from build123d import *

# Parameters (mm, degrees)
SKETCH1_W                        = 156
SKETCH1_H                        = 260
BOSS_EXTRUDE1_DEPTH              = 10
BOSS_EXTRUDE2_DEPTH              = 66
SKETCH3_R                        = 40
CUT_EXTRUDE1_DEPTH               = 77
SKETCH4_W                        = 20
SKETCH4_H                        = 37.5
CUT_EXTRUDE2_DEPTH               = 5
SKETCH6_W                        = 15
SKETCH6_H                        = 15
BOSS_EXTRUDE3_DEPTH              = 10
SKETCH7_R                        = 4
CUT_EXTRUDE4_DEPTH               = 10
FILLET1_R                        = 2
SKETCH8_W                        = 156
SKETCH8_H                        = 10
BOSS_EXTRUDE4_DEPTH              = 10
SKETCH9_R                        = 4
CUT_EXTRUDE5_DEPTH               = 77
SKETCH10_W                       = 156
SKETCH10_H                       = 10
BOSS_EXTRUDE5_DEPTH              = 25
SKETCH11_W                       = 28
SKETCH11_H                       = 295
BOSS_EXTRUDE6_DEPTH              = 10
BOSS_EXTRUDE7_DEPTH              = 212
SKETCH13_R                       = 3
CUT_EXTRUDE6_DEPTH               = 11
BOSS_EXTRUDE10_DEPTH             = 212
SKETCH18_R                       = 3
CUT_EXTRUDE8_DEPTH               = 11
SKETCH19_R                       = 10
CUT_EXTRUDE9_DEPTH               = 113
BOSS_EXTRUDE11_REACH             = 47.35
SKETCH20_W                       = 10
SKETCH20_H                       = 86
BOSS_EXTRUDE11_DIRECTION_2_REACH = 366.652
FILLET2_R                        = 20
SKETCH21_R                       = 15
CUT_EXTRUDE11_DEPTH              = 5
SKETCH22_W                       = 30
SKETCH22_H                       = 20
CUT_EXTRUDE12_DEPTH              = 1
CUT_EXTRUDE12_DEPTH_BACK         = 213
SKETCH23_W                       = 40
SKETCH23_H                       = 6.35
CUT_EXTRUDE13_DEPTH              = 1
CUT_EXTRUDE13_DEPTH_BACK         = 213


with BuildPart() as part:
    # Sketch1 → Boss-Extrude1 (new body)
    with BuildSketch(Plane(origin=(0, 0, 0), x_dir=(1, 0, 0), z_dir=(0, 1, 0))):
        Rectangle(SKETCH1_W, SKETCH1_H)
    extrude(amount=BOSS_EXTRUDE1_DEPTH)

    # Sketch2 → Boss-Extrude2 (add)
    with BuildSketch(Plane.XZ):
        Polygon((-73, -120), (-73, 125), (73, 125), (73, -120), (78, -120), (78, 130), (-78, 130), (-78, -120), align=None)
    extrude(amount=BOSS_EXTRUDE2_DEPTH)

    # Sketch3 → Cut-Extrude1 (cut, through all)
    with BuildSketch(Plane(origin=(0, 10, 0), x_dir=(1, 0, 0), z_dir=(0, 1, 0))):
        with Locations((0, -70)):
            Circle(SKETCH3_R)
    extrude(amount=-CUT_EXTRUDE1_DEPTH, mode=Mode.SUBTRACT)

    # Sketch4 → Cut-Extrude2 (cut)
    with BuildSketch(Plane.XY.offset(130)):
        with Locations((-62.5, -47.25)):
            Rectangle(SKETCH4_W, SKETCH4_H)
        with Locations((62.5, -47.25)):
            Rectangle(SKETCH4_W, SKETCH4_H)
    extrude(amount=-CUT_EXTRUDE2_DEPTH, mode=Mode.SUBTRACT)

    # Sketch6 → Boss-Extrude3 (add)
    with BuildSketch(Plane.XZ.offset(66)):
        with Locations((0, 137.5)):
            Rectangle(SKETCH6_W, SKETCH6_H)
    extrude(amount=-BOSS_EXTRUDE3_DEPTH)

    # Sketch7 → Cut-Extrude4 (cut)
    with BuildSketch(Plane.XZ.offset(66)):
        with Locations((0, 137.5)):
            Circle(SKETCH7_R)
    extrude(amount=-CUT_EXTRUDE4_DEPTH, mode=Mode.SUBTRACT)

    # Fillet1
    fillet1_edges = [part.edges().sort_by_distance(p)[0] for p in [
        (7.5, -61, 145),
        (-7.5, -61, 145),
    ]]
    fillet(fillet1_edges, radius=FILLET1_R)

    # Sketch8 → Boss-Extrude4 (add)
    with BuildSketch(Plane(origin=(0, 0, -130), x_dir=(-1, 0, 0), z_dir=(0, 0, -1))):
        with Locations((0, 5)):
            Rectangle(SKETCH8_W, SKETCH8_H)
    extrude(amount=BOSS_EXTRUDE4_DEPTH)

    # Sketch9 → Cut-Extrude5 (cut, through all)
    with BuildSketch(Plane(origin=(0, 10, 0), x_dir=(1, 0, 0), z_dir=(0, 1, 0))):
        with Locations((-68, 130)):
            Circle(SKETCH9_R)
        with Locations((68, 130)):
            Circle(SKETCH9_R)
    extrude(amount=-CUT_EXTRUDE5_DEPTH, mode=Mode.SUBTRACT)

    # Sketch10 → Boss-Extrude5 (add)
    with BuildSketch(Plane(origin=(0, 0, -140), x_dir=(-1, 0, 0), z_dir=(0, 0, -1))):
        with Locations((0, 5)):
            Rectangle(SKETCH10_W, SKETCH10_H)
    extrude(amount=BOSS_EXTRUDE5_DEPTH)

    # Sketch11 → Boss-Extrude6 (add)
    with BuildSketch(Plane(origin=(0, 10, 0), x_dir=(1, 0, 0), z_dir=(0, 1, 0))):
        with Locations((-92, 17.5)):
            Rectangle(SKETCH11_W, SKETCH11_H)
        with Locations((92, 17.5)):
            Rectangle(SKETCH11_W, SKETCH11_H)
    extrude(amount=-BOSS_EXTRUDE6_DEPTH)

    # Sketch12 → Boss-Extrude7 (add)
    with BuildSketch(Plane.ZY.offset(106)):
        Polygon((-165, 0), (-190.349999035, -86), (-210.349999035, -86), (-210.349999035, -76), (-190.349999035, -76), (-165, 10), align=None)
    extrude(amount=-BOSS_EXTRUDE7_DEPTH)

    # Sketch13 → Cut-Extrude6 (cut, through all)
    with BuildSketch(Plane(origin=(0, -76, 0), x_dir=(1, 0, 0), z_dir=(0, 1, 0))):
        with Locations((-96, 200.349999035)):
            Circle(SKETCH13_R)
        with Locations((96, 200.349999035)):
            Circle(SKETCH13_R)
    extrude(amount=-CUT_EXTRUDE6_DEPTH, mode=Mode.SUBTRACT)

    # Sketch17 → Boss-Extrude10 (add)
    with BuildSketch(Plane(origin=(106, 0, 0), x_dir=(0, 0, -1), z_dir=(1, 0, 0))):
        Polygon((-130, 0), (-179.65212315, -86), (-199.65212315, -86), (-199.65212315, -76), (-179.65212315, -76), (-130, 10), align=None)
    extrude(amount=-BOSS_EXTRUDE10_DEPTH)

    # Sketch18 → Cut-Extrude8 (cut, through all)
    with BuildSketch(Plane(origin=(0, -76, 0), x_dir=(1, 0, 0), z_dir=(0, 1, 0))):
        with Locations((-96, -189.65212315)):
            Circle(SKETCH18_R)
        with Locations((96, -189.65212315)):
            Circle(SKETCH18_R)
    extrude(amount=-CUT_EXTRUDE8_DEPTH, mode=Mode.SUBTRACT)

    # Sketch19 → Cut-Extrude9 (cut)
    with BuildSketch(Plane.XY.offset(130)):
        with Locations((-62.5, -38.5)):
            Circle(SKETCH19_R)
        with Locations((62.5, -38.5)):
            Circle(SKETCH19_R)
    extrude(amount=CUT_EXTRUDE9_DEPTH, mode=Mode.SUBTRACT)

    # Boss-Extrude11: up to this face of the body (flat: up to its plane)
    boss_extrude11_end = Plane(part.part.faces().sort_by_distance((0, -33, -177.674999518))[0])
    # Sketch20 → Boss-Extrude11 (add, up to the picked face)
    with BuildSketch(Plane(origin=(0, 0, -165), x_dir=(-1, 0, 0), z_dir=(0, 0, -1)), mode=Mode.PRIVATE) as boss_extrude11_sk1:
        with Locations((-101, -43)):
            Rectangle(SKETCH20_W, SKETCH20_H)
    boss_extrude11_tool1 = split(extrude(boss_extrude11_sk1.sketch, amount=BOSS_EXTRUDE11_REACH, mode=Mode.PRIVATE), bisect_by=boss_extrude11_end, keep=Keep.BOTH, mode=Mode.PRIVATE)
    add(boss_extrude11_tool1.solids().sort_by_distance((101, -43, -165))[0])
    # Sketch20 → Boss-Extrude11 (add, up to the picked face)
    with BuildSketch(Plane(origin=(0, 0, -165), x_dir=(-1, 0, 0), z_dir=(0, 0, -1)), mode=Mode.PRIVATE) as boss_extrude11_sk2:
        with Locations((101, -43)):
            Rectangle(SKETCH20_W, SKETCH20_H)
    boss_extrude11_tool2 = split(extrude(boss_extrude11_sk2.sketch, amount=BOSS_EXTRUDE11_REACH, mode=Mode.PRIVATE), bisect_by=boss_extrude11_end, keep=Keep.BOTH, mode=Mode.PRIVATE)
    add(boss_extrude11_tool2.solids().sort_by_distance((-101, -43, -165))[0])

    # Sketch20 → Boss-Extrude11 direction 2 (add, up to next)
    with BuildSketch(Plane(origin=(0, 0, -165), x_dir=(-1, 0, 0), z_dir=(0, 0, -1)), mode=Mode.PRIVATE) as boss_extrude11_direction_2_sk1:
        with Locations((-101, -43)):
            Rectangle(SKETCH20_W, SKETCH20_H)
    boss_extrude11_direction_2_tool1 = extrude(boss_extrude11_direction_2_sk1.sketch, amount=-BOSS_EXTRUDE11_DIRECTION_2_REACH, mode=Mode.PRIVATE) - part.part
    add(boss_extrude11_direction_2_tool1.solids().sort_by_distance((101, -43, -165))[0])
    # Sketch20 → Boss-Extrude11 direction 2 (add, up to next)
    with BuildSketch(Plane(origin=(0, 0, -165), x_dir=(-1, 0, 0), z_dir=(0, 0, -1)), mode=Mode.PRIVATE) as boss_extrude11_direction_2_sk2:
        with Locations((101, -43)):
            Rectangle(SKETCH20_W, SKETCH20_H)
    boss_extrude11_direction_2_tool2 = extrude(boss_extrude11_direction_2_sk2.sketch, amount=-BOSS_EXTRUDE11_DIRECTION_2_REACH, mode=Mode.PRIVATE) - part.part
    add(boss_extrude11_direction_2_tool2.solids().sort_by_distance((-101, -43, -165))[0])

    # Fillet2
    fillet2_edges = [part.edges().sort_by_distance(p)[0] for p in [
        (0, 10, -165),
        (0, 10, 130),
    ]]
    fillet(fillet2_edges, radius=FILLET2_R)

    # Sketch21 → Cut-Extrude11 (cut)
    with BuildSketch(Plane(origin=(78, 0, 0), x_dir=(0, 0, -1), z_dir=(1, 0, 0))):
        with Locations((90, -30.5)):
            Circle(SKETCH21_R)
    extrude(amount=-CUT_EXTRUDE11_DEPTH, mode=Mode.SUBTRACT)

    # Sketch22 → Cut-Extrude12 (cut, two sides)
    with BuildSketch(Plane(origin=(106, 0, 0), x_dir=(0, 0, -1), z_dir=(1, 0, 0))) as cut_extrude12_sk:
        with Locations((-105, -76)):
            Rectangle(SKETCH22_W, SKETCH22_H)
        with Locations((49.5, -76)):
            Rectangle(SKETCH22_W, SKETCH22_H)
    extrude(amount=CUT_EXTRUDE12_DEPTH, mode=Mode.SUBTRACT)
    extrude(cut_extrude12_sk.sketch, amount=-CUT_EXTRUDE12_DEPTH_BACK, mode=Mode.SUBTRACT)

    # Sketch23 → Cut-Extrude13 (cut, two sides)
    with BuildSketch(Plane.ZY.offset(106)) as cut_extrude13_sk:
        with Locations((-102.849999035, -82.825)):
            Rectangle(SKETCH23_W, SKETCH23_H)
        with Locations((92.150000965, -82.825)):
            Rectangle(SKETCH23_W, SKETCH23_H)
    extrude(amount=CUT_EXTRUDE13_DEPTH, mode=Mode.SUBTRACT)
    extrude(cut_extrude13_sk.sketch, amount=-CUT_EXTRUDE13_DEPTH_BACK, mode=Mode.SUBTRACT)


solid = part.part
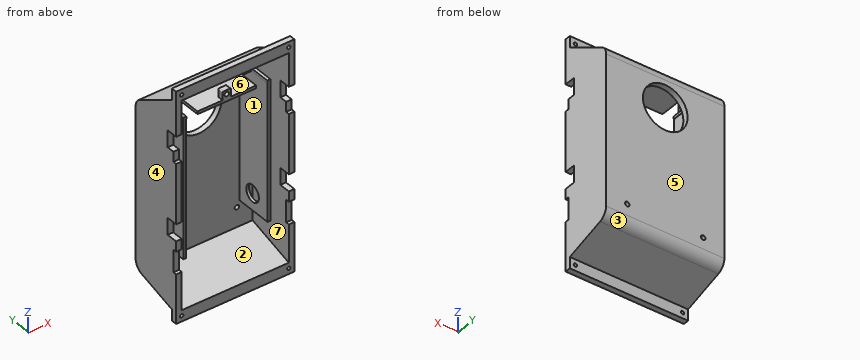
CAD build for the part. Positions are in the model's coordinates, mm. Face numbers are marked on the shaded views. A direction names the side the tool comes from. Give positions to 0.01 mm unless a question says otherwise; leave off trailing zeros. Write each loop counter-clockwise with the first axis right and the second up, starting at its lowest first coordinate (ties: lowest second). Pieces come first, ordered by that corner, then holes. Notation, with made-up numbers: (48, -27) - (81, -27) arc R10 ccw to (81, -12) - close; hole circle Ø3 at (17, 53). An arc over 180 degrees is marked (long way). Answer as CSV lines item,"result".
Q1. Drill centre lines: line 1 (X direction, y = -55, z = -8.5); line 2 (Z direction, x = -75.5, y = -47); line 3 (X direction, y = -61, z = 137). Where is each one in solid material? Low to high. Write a range as from..to.
Result set:
line 1,"-106..-96, -78..-73, 73..78, 96..106"
line 2,"-181.8..-178.85, -120..130, 157.14..162.91"
line 3,"-106..-96, -7.5..-3.97, 3.97..7.5, 96..106"
Q2. Flat gauge pins, fed straight in: pin 1 Ø8 at (x, z) = (99.5, 112) entering from -Y; pin 2 Ø3 at (x, z) = (48.5, -154.5) entering from +Y; pin 3 Ø18 at (x, y) = (62.5, -38.5) entering from -Z. Where does each tip first touch, or does it go through?
Result set:
pin 1,"y = -66"
pin 2,"y = 9.78"
pin 3,"z = -181.95"
Q3. Band-saw the part on D-D (z = -25). Give the cut face in (x, y), and give its area (3 significant figures).
Result set:
outline,"(-106, -86) - (-96, -86) - (-96, 0) - (-78, 0) - (-78, -66) - (-73, -66) - (-73, 0) - (73, 0) - (73, -66) - (78, -66) - (78, 0) - (96, 0) - (96, -86) - (106, -86) - (106, 10) - (-106, 10) - close"
area,"4,500 mm²"
Q4. Pull direction X, two halves, no side cores. Call the marked faces 1, 2, 3 and 4: released by +X, released by -X, zero draft, split by the parting line, or undercut.
Result set:
face 1,"undercut"
face 2,"undercut"
face 3,"zero draft"
face 4,"released by -X"
Q5. Band-saw the part on A-A (z = -90). Give the cut face in (x, y).
Result set:
outline,"(-106, -79.65) - (-96, -79.65) - (-96, 0) - (-78, 0) - (-78, -66) - (-73, -66) - (-73, 0) - (73, 0) - (73, -15.5) - (78, -15.5) - (78, 0) - (96, 0) - (96, -79.65) - (106, -79.65) - (106, 10) - (-106, 10) - close; (73, -66) - (78, -66) - (78, -45.5) - (73, -45.5) - close"
Q6. 3-axis set-ups, long thin cutter, end or side, ignore diameter. For the marked faces 5, 6 and 7: which of +Z, -Z, +X, -X, +Y, -Y reach the whole face in a straight line?
Result set:
face 5,"+Z, -Z, +X, -X, +Y"
face 6,"none"
face 7,"-Y"
Q7. Band-saw the part on B-B (y = -8.5). Give the cut face in (x, z), and give its area (3 significant figures).
Result set:
outline,"(-106, -170.45) - (106, -170.45) - (106, 140.68) - (-106, 140.68) - close; (-78, -120) - (-73, -120) - (-73, 125) - (73, 125) - (73, -120) - (78, -120) - (78, 130) - (-78, 130) - close; hole (-96, -167.51) - (96, -167.51) - (96, 134.91) - (-96, 134.91) - close"
area,"11,100 mm²"
Q8. Band-saw the part on C-C (x = 0). Give the cut face in (y, z), and give its area (3 significant figures).
Result set:
outline,"(-86, -210.35) - (-76, -210.35) - (-76, -190.35) - (-4.35, -169.23) arc R20 ccw to (10, -150.04) - (10, 30) - (0, 30) - (0, -165) - (-86, -190.35) - close; (-86, 179.65) - (0, 130) - (-56, 130) - (-56, 133.5) - (-66, 133.5) - (-66, 125) - (0, 125) - (0, 110) - (10, 110) - (10, 118.45) arc R20 ccw to (0, 135.77) - (-76, 179.65) - (-76, 199.65) - (-86, 199.65) - close; (-66, 141.5) - (-56, 141.5) - (-56, 145) - (-66, 145) - close"
area,"3,640 mm²"
